```python
from build123d import *

# Parameters (mm, degrees)
SKETCH_1_R      = 2
SKETCH_1_R_2    = 25
SKETCH_1_R_3    = 2.05
SKETCH_1_R_4    = 2.1
SKETCH_1_W      = 8.1
SKETCH_1_H      = 2.1
SKETCH_1_W_2    = 8.2
SKETCH_1_W_3    = 2.2
SKETCH_1_H_2    = 8.2
EXTRUDE_1_DEPTH = 2
FILLET_2_R      = 2


with BuildPart() as part:
    # 草图1 → 凸台-拉伸1 (new body)
    with BuildSketch(Plane.XY):
        Polygon((7.027428163, -4.999036262), (20.810808237, -16.956988843), (73.227648339, -16.964389058), (87.027428163, -16.964389058), (87.027428163, 75.054738201), (67.497807203, 94.584359161), (63.997628636, 91.084180595), (62.512704395, 89.599256354), (56.785139468, 95.326821282), (58.270063708, 96.811745522), (61.771734574, 100.31043179), (54.027428163, 108.054738201), (46.284614051, 115.797552313), (42.784435485, 112.297373746), (41.299511244, 110.812449505), (35.571946316, 116.540014433), (37.056870557, 118.024938674), (40.557049124, 121.52511724), (21.027428163, 141.054738201), (-114.884210676, 141.054738201), (-121.955278488, 123.983670389), (-100.755816342, 102.784208243), (-97.257364322, 106.282660262), (-95.772440082, 107.767584503), (-90.044875154, 102.040019575), (-91.529799395, 100.555095335), (-95.028251414, 97.056643315), (-87.28543216, 89.313824061), (-79.542612906, 81.571004807), (-76.044160887, 85.069456827), (-74.559236646, 86.554381067), (-68.831671719, 80.82681614), (-70.316595959, 79.341891899), (-73.815047978, 75.84343988), align=None)
        with Locations((-52.972571837, 135.054738201)):
            Circle(SKETCH_1_R, mode=Mode.SUBTRACT)
        with Locations((47.027428163, 15.054738201)):
            Circle(SKETCH_1_R_2, mode=Mode.SUBTRACT)
        with Locations(Location((-22.972571837, 135.054738201, 0), (0, 0, 180))):
            Circle(SKETCH_1_R, mode=Mode.SUBTRACT)
        with Locations((7.027428163, 135.054738201)):
            Circle(SKETCH_1_R, mode=Mode.SUBTRACT)
        with Locations(Location((-112.972571837, 135.054738201, 0), (0, 0, 180))):
            Circle(SKETCH_1_R, mode=Mode.SUBTRACT)
        with Locations((-82.972571837, 135.054738201)):
            Circle(SKETCH_1_R, mode=Mode.SUBTRACT)
        with Locations((49.784787476, 103.812097514)):
            Circle(SKETCH_1_R, mode=Mode.SUBTRACT)
        with Locations((-83.04451802, 93.554738201)):
            Circle(SKETCH_1_R, mode=Mode.SUBTRACT)
        with Locations((20.275835807, 57.054738201)):
            Circle(SKETCH_1_R_3, mode=Mode.SUBTRACT)
        with Locations((-6.58531727, 99.226748532)):
            Circle(SKETCH_1_R_3, mode=Mode.SUBTRACT)
        with Locations((70.527428163, -8.445261799)):
            Circle(SKETCH_1_R_4, mode=Mode.SUBTRACT)
        with Locations((23.527428163, -8.445261799)):
            Circle(SKETCH_1_R_4, mode=Mode.SUBTRACT)
        with Locations((23.527428163, 38.554738201)):
            Circle(SKETCH_1_R_4, mode=Mode.SUBTRACT)
        with Locations((70.527428163, 38.554738201)):
            Circle(SKETCH_1_R_4, mode=Mode.SUBTRACT)
        with Locations((81.392055944, 72.204829046)):
            Circle(SKETCH_1_R_3, mode=Mode.SUBTRACT)
        with Locations((81.392055944, -8.445261799)):
            Circle(SKETCH_1_R_3, mode=Mode.SUBTRACT)
        with Locations((81.392055944, 42.204829046)):
            Circle(SKETCH_1_R_3, mode=Mode.SUBTRACT)
        with Locations((-37.972571837, 135.054738201)):
            Rectangle(SKETCH_1_W, SKETCH_1_H, mode=Mode.SUBTRACT)
        with Locations((-7.972571837, 135.054738201)):
            Rectangle(SKETCH_1_W, SKETCH_1_H, mode=Mode.SUBTRACT)
        with Locations((-97.972571837, 135.054738201)):
            Rectangle(SKETCH_1_W, SKETCH_1_H, mode=Mode.SUBTRACT)
        with Locations((-67.972571837, 135.054738201)):
            Rectangle(SKETCH_1_W, SKETCH_1_H, mode=Mode.SUBTRACT)
        with Locations((5.275835807, 57.054738201)):
            Rectangle(SKETCH_1_W_2, SKETCH_1_H, mode=Mode.SUBTRACT)
        with Locations((35.275835807, 57.054738201)):
            Rectangle(SKETCH_1_W_2, SKETCH_1_H, mode=Mode.SUBTRACT)
        Polygon((-26.317798475, 106.3059132), (-58.783300448, 90.506724064), (-82.786741677, 114.510165293), (-76.96930946, 120.054738201), (-32.606331473, 120.054738201), align=None, mode=Mode.SUBTRACT)
        Polygon((47.299709176, 85.219712632), (24.92619293, 73.952191934), (4.862626833, 105.451990707), (-2.731253041, 122.054738201), (2.37892986, 122.054738201), align=None, mode=Mode.SUBTRACT)
        Polygon((-14.950211349, 60.939664471), (-17.845757969, 77.065019133), (-38.30861977, 67.106860342), (-24.982934729, 50.626518371), align=None, mode=Mode.SUBTRACT)
        Polygon((2.01437662, 34.262984309), (13.802642778, 20.368597473), (13.802642778, 31.594822975), align=None, mode=Mode.SUBTRACT)
        with Locations((81.392055944, 57.204829046)):
            Rectangle(SKETCH_1_W_3, SKETCH_1_H_2, mode=Mode.SUBTRACT)
        with Locations((81.392055944, 6.554738201)):
            Rectangle(SKETCH_1_W_3, SKETCH_1_H_2, mode=Mode.SUBTRACT)
    extrude(amount=EXTRUDE_1_DEPTH)

    # 圆角2
    fillet_2_edges = [part.edges().sort_by_distance(p)[0] for p in [
        (-26.317798475, 106.3059132, 1),
        (-32.606331473, 120.054738201, 1),
        (-76.96930946, 120.054738201, 1),
        (-82.786741677, 114.510165293, 1),
        (-58.783300448, 90.506724064, 1),
        (47.299709176, 85.219712632, 1),
        (2.37892986, 122.054738201, 1),
        (-2.731253041, 122.054738201, 1),
        (24.92619293, 73.952191934, 1),
        (-24.982934729, 50.626518371, 1),
        (-14.950211349, 60.939664471, 1),
        (-17.845757969, 77.065019133, 1),
        (-38.30861977, 67.106860342, 1),
        (13.802642778, 31.594822975, 1),
        (2.01437662, 34.262984309, 1),
        (13.802642778, 20.368597473, 1),
        (40.557049124, 121.52511724, 1),
        (46.284614051, 115.797552313, 1),
        (61.771734574, 100.31043179, 1),
        (67.497807203, 94.584359161, 1),
        (87.027428163, -16.964389058, 1),
        (-73.815047978, 75.84343988, 1),
        (-79.542612906, 81.571004807, 1),
        (-95.028251414, 97.056643315, 1),
        (-100.755816342, 102.784208243, 1),
        (-121.955278488, 123.983670389, 1),
        (-114.884210676, 141.054738201, 1),
    ]]
    fillet(fillet_2_edges, radius=FILLET_2_R)


solid = part.part
```
The listing builds one solid part. Answer for the finished solid, in the listing's coordinates (mm). A direction names the side the tool comes from. Give positions to 0.01 mm unless a question says otherwise; leave off trailing zeros. Order: outer loops, then holes, each group sorted by start corner. A loop starts at its lowest first (then second) coordinate and runs counter-clockwise, first axis right, second up. Notation, with made-up numbers: (70.5, 18.25) -> (77.5, 18.25) arc R36 cw to (77.5, 56.25) -> close; hole circle Ø2 at (42.5, -22). An arc over 180 degrees is marked (long way). Answer as a JSON object with one key per item and string values. Group by question number.
Item 1: The part is cut by section A-A on y = -2. Write down the section's boundary in (x, z), and give its area (3 significant figures).
Item 2: Flat-ended cylindrical pins translate along their axes: pin 1 (1 mm diameter, centred on x = -83, z = 1, fed in from -Y); pin 2 (1 mm diameter, centred on x = 81.5, z = 1, fed in from +Y); pin 3 (3.5 mm diameter, centred on x = -112.97, y = 135.05, fed in from +Z). Find the tip coordinate at first contact, or state that the pin passes through.
Item 3: The part is cut by section B-B on z = 1.4. Give the number of separate pieces and of enclosed holes in the cut face, and give its area (3 significant figures).
Item 4: Consider L1, parallel to Y at x = 24, z = 1; L2, parallel to Y at x = 31.5, z = 0.25; L3, parallel to X at y = 37.5, z = 1.55. Determine where each line is inside the solid, lowest interval first. Write a range as from..to.
Item 5: Determine the mould class of faces 1 (the flat face through (54.116, 107.966, 0.986)), 2 (the flat face through (-31.636, 58.855, 0.986)), 3 (the flat face through (-87.37, 89.4, 0.99)) for opening direction X: pulls with the +X half, pulls with the -X half, needs draft (parallel to the pull), parting line crosses it, or undercut.
Item 6: A tool of negligible diameter and unlimited length cuts with its end or side. For faces 4 (the flat face through (-70.414, 102.137, 0.986)), 5 (the flat face through (30.21, 131.87, 0.99)), from which of +Z, -Z, +X, -X, +Y, -Y can it reach the whole face along a straight path? Write none if from no direction.
Item 7: The part is cut by section C-C on y = 130.5. Write down the section's boundary in (x, z), and give its area (3 significant figures).
Result set:
{
 "1": {"outline": "(4.03, 0) -> (28.75, 0) -> (28.75, 2) -> (4.03, 2) -> close; (65.31, 0) -> (87.03, 0) -> (87.03, 2) -> (65.31, 2) -> close", "area": "92.9 mm²"},
 "2": {"pin 1": "y = 84.53", "pin 2": "y = 81.08", "pin 3": "through"},
 "3": {"separate pieces": "1", "enclosed holes": "29", "area": "16,000 mm²"},
 "4": {"L1": "-16.96..-10.49, -6.4..5.32, 24.79..36.51, 40.6..75.41, 104.33..138.08", "L2": "-16.96..-4.54, 34.65..56, 58.1..77.26, 98.18..130.58", "L3": "-35.47..21.71, 25.34..36.02, 58.04..68.71, 72.34..87.03"},
 "5": {"face 1": "pulls with the +X half", "face 2": "undercut", "face 3": "pulls with the -X half"},
 "6": {"face 4": "+Z, -Z", "face 5": "+Z, -Z, +X, +Y"},
 "7": {"outline": "(-119.26, 0) -> (31.58, 0) -> (31.58, 2) -> (-119.26, 2) -> close", "area": "302 mm²"}
}
